Input: part model. Units: mm. Frame: model coordinates. A direction names the side the tool comes from. Round coordinates to 2 decimals unless told otherwise and drop trailing zeros. Write each loop counter-clockwise with the first axis right and the second up, starting at its lowest first coordinate (ties: lowest second). Pieces come first, ordered by that corner, then holes. Notation, with made-up numbers: M -16,52 L 43,52 A19 ccw 43,80 Z; hole C 26.5,79.25 d7. An arc over 180 degrees is marked long. Answer as CSV lines item,"result". Start each with the question number.
```python
from build123d import *

# Parameters (mm, degrees)
SKETCH1_W           = 26
SKETCH1_H           = 18
BOSS_EXTRUDE1_DEPTH = 13
SKETCH2_R           = 1.35
SKETCH2_W           = 16.5
SKETCH2_H           = 3.5
CUT_EXTRUDE1_DEPTH  = 14


with BuildPart() as part:
    # Sketch1 → Boss-Extrude1 (new body)
    with BuildSketch(Plane(origin=(0, 0, 0), x_dir=(1, 0, 0), z_dir=(0, 1, 0))):
        with Locations((13, 9)):
            Rectangle(SKETCH1_W, SKETCH1_H)
    extrude(amount=BOSS_EXTRUDE1_DEPTH)

    # Sketch2 → Cut-Extrude1 (cut, through all)
    with BuildSketch(Plane(origin=(0, 13, 0), x_dir=(1, 0, 0), z_dir=(0, 1, 0))):
        with Locations((3, 15.25)):
            Circle(SKETCH2_R)
        with Locations((23, 15.25)):
            Circle(SKETCH2_R)
        with Locations((3, 2.75)):
            Circle(SKETCH2_R)
        with Locations((23, 2.75)):
            Circle(SKETCH2_R)
        with Locations((13, 15.25)):
            Rectangle(SKETCH2_W, SKETCH2_H)
        with Locations((13, 2.75)):
            Rectangle(SKETCH2_W, SKETCH2_H)
    extrude(amount=-CUT_EXTRUDE1_DEPTH, mode=Mode.SUBTRACT)


solid = part.part
```
Item 1: Cut plane D-D, the plane x = 15.5. Return loops of the section in (y, z), plus the area to 3 significant figures.
Item 2: Cut plane A-A, the plane x = 23. Return loops of the section in (y, z).
Item 3: Cut plane B-B, the plane z = -2.75. Return loops of the section in (x, y), plus the area to 3 significant figures.
Item 4: Access query for faces 1 (the face through (13, 6, -18)), 2 (the face through (4.75, 7, -3)). Directions: +Z, -Z, +X, -X, +Y, -Y. A direction counts if a zero-diameter tool reaches every point of the face in a straight line with its end or side. Return the directions, or none.
Item 5: Draft query along X for faces 3 (the face through (21.25, 7, -15)), 4 (the face through (0, 6, -9)), 5 (the face through (13, 13, -9)). Return one class per face: +X half, -X half, draft (parallel to the pull), parting line (faces both ways), or undercut.
Item 6: Cut plane C-C, the plane y = 2.25. Return loops of the section in (x, z), plus the area to 3 significant figures.
Item 7: Line query: line 1 (Z direction, x = 3, y = 8); line 2 (Z direction, x = 5.5, y = 3.75); line 3 (X direction, y = 3.75, z = -2.75). Output: solid intervals per line, ascending. Write a range as [from, to].
Results list:
1,outline,"M 0,-18 L 13,-18 L 13,-17 L 0,-17 Z; M 0,-13.5 L 13,-13.5 L 13,-4.5 L 0,-4.5 Z; M 0,-1 L 13,-1 L 13,0 L 0,0 Z"
1,area,"143 mm²"
2,outline,"M 0,-18 L 13,-18 L 13,-16.6 L 0,-16.6 Z; M 0,-13.9 L 13,-13.9 L 13,-4.1 L 0,-4.1 Z; M 0,-1.4 L 13,-1.4 L 13,0 L 0,0 Z"
3,outline,"M 0,0 L 1.65,0 L 1.65,13 L 0,13 Z; M 4.35,0 L 4.75,0 L 4.75,13 L 4.35,13 Z; M 21.25,0 L 21.65,0 L 21.65,13 L 21.25,13 Z; M 24.35,0 L 26,0 L 26,13 L 24.35,13 Z"
3,area,"53.3 mm²"
4,face 1,"-Z, +X, -X, +Y, -Y"
4,face 2,"+Y, -Y"
5,face 3,"undercut"
5,face 4,"-X half"
5,face 5,"draft"
6,outline,"M 0,-18 L 26,-18 L 26,0 L 0,0 Z; hole C 3,-15.25 d2.7; hole C 3,-2.75 d2.7; hole M 4.75,-17 L 21.25,-17 L 21.25,-13.5 L 4.75,-13.5 Z; hole M 4.75,-4.5 L 21.25,-4.5 L 21.25,-1 L 4.75,-1 Z; hole C 23,-15.25 d2.7; hole C 23,-2.75 d2.7"
6,area,"330 mm²"
7,line 1,"[-18, -16.6], [-13.9, -4.1], [-1.4, 0]"
7,line 2,"[-18, -17], [-13.5, -4.5], [-1, 0]"
7,line 3,"[0, 1.65], [4.35, 4.75], [21.25, 21.65], [24.35, 26]"
